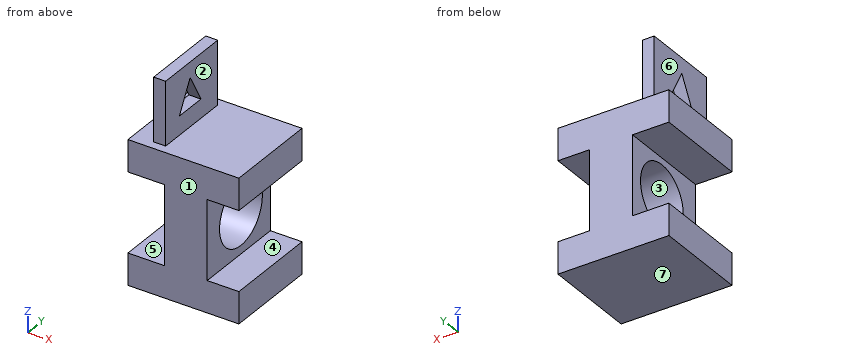
```python
from build123d import *

# Parameters (mm, degrees)
F1_DEPTH = 76.2
F2_W     = 9.595008567
F2_H     = 62.8318372183
F3_DEPTH = 50.8
F5_DEPTH = 25.5704986105
F6_R     = 25.7972308172
F7_DEPTH = 59.7263876276


with BuildPart() as f1:
    # F0 (on Front) → F1 (new body)
    with BuildSketch(Plane.XZ):
        Polygon((-44.6047578722, -25.4), (-44.6047578722, -50.8), (44.2952421278, -50.8), (44.2952421278, -25.4), (18.8952421278, -25.4), (18.8952421278, 38.1), (44.2952421278, 38.1), (44.2952421278, 63.5), (-44.6047578722, 63.5), (-44.6047578722, 38.1), (-15.4301454999, 38.1), (-15.4301454999, -25.4), align=None)
    extrude(amount=F1_DEPTH)

    # F2 (on face) → F3 (join)
    with BuildSketch(Plane.XY.offset(63.5)):
        with Locations((-23.8327635452, -37.7904830966)):
            Rectangle(F2_W, F2_H)
    extrude(amount=F3_DEPTH)

    # F4 (on face) → F5 (cut, through all)
    with BuildSketch(Plane.YZ.offset(-19.0352592617)):
        Polygon((-52.6472702622, 78.5312056541), (-26.647888124, 78.5312056541), (-39.6475791931, 102.0544543862), align=None)
    extrude(amount=-F5_DEPTH, mode=Mode.SUBTRACT)

    # F6 (on face) → F7 (cut, through all)
    with BuildSketch(Plane(origin=(-15.4301454999, 0, 0), x_dir=(0, -1, 0), z_dir=(-1, 0, 0))):
        with Locations((35.4866050184, 7.0887273178)):
            Circle(F6_R)
    extrude(amount=-F7_DEPTH, mode=Mode.SUBTRACT)


solid = f1.part
```
Could you check a few things on this model? Use its own coordinates, in mm. Face numbers are marked on the shaded views. A direction names the side the tool comes from. Coordinates: 2 decimals unless noted, no trailing zeros. Order: outer loops, then holes, each group sorted by start corner. A loop starts at its lowest first (then second) coordinate and runs counter-clockwise, first axis right, second up. Notation, with made-up numbers: M -35.75,-40 L -6.75,-40 A27 ccw -6.75,-19 Z; hole C -25.5,82 d3. An arc over 180 degrees is marked long. Use a Markdown table: item, result. Add a question column.
Q1. I want a section at A-A on x = -24. List the corners of the cut face in (y, z) for me, then the cut area to 3 significant figures.
Q2. I want a section at D-D on y = -42.5. List the corners of the cut face in (x, z) for me, then the cut area to 3 significant figures.
Q3. If I drill on L1, parallel to Z at x = -31, y = -57; L2, parallel to Z at x = -2.5, y = -36; L3, parallel to X at y = -44.5, z = 33.5, over which ranges is the centre line in solid material (lowest first)?
Q4. Which directions (+Z, -Z, +X, -X, +Y, -Y) give clear straight access to the entire face, cutting with the end or side of a thin tool? Please do the marked faces 4, 5, 6 and 7.
Q5. I want a section at C-C on z = 21.5. List the corners of the cut face in (x, y) for me, then the cut area to 3 significant figures.
Q6. I want a section at B-B on x = 25. List the corners of the cut face in (y, z) for me.
Q7. I'm going to push flat-ended pins straight in: pin 1 (6 mm diameter, centred on y = -25, z = -22, fed in from -X); pin 2 (1 mm diameter, centred on x = 21, y = -29.5, fed in from +Z); pin 3 (10.5 mm diameter, centred on x = -24, z = 88.5, fed in from +Y). Where does each tip first touch, or does it pass through?
Q8. We'd pull the mould along Y, two halves only. Please class the marked faces 1, 2 and 3: pulls with the +Y half, pulls with the -Y half, needs draft (parallel to the pull), parting line crosses it, or undercut.
Checked values:
| question | item | result |
|---|---|---|
| 1 | outline | M -76.2,-50.8 L 0,-50.8 L 0,-25.4 L -76.2,-25.4 Z; M -76.2,38.1 L 0,38.1 L 0,63.5 L -6.37,63.5 L -6.37,114.3 L -69.21,114.3 L -69.21,63.5 L -76.2,63.5 Z; hole M -52.65,78.53 L -26.65,78.53 L -39.65,102.05 Z |
| 1 | area | 6,760 mm² |
| 2 | outline | M -44.6,-50.8 L 44.3,-50.8 L 44.3,-25.4 L 18.9,-25.4 L 18.9,-17.74 L -15.43,-17.74 L -15.43,-25.4 L -44.6,-25.4 Z; M -44.6,38.1 L -15.43,38.1 L -15.43,31.91 L 18.9,31.91 L 18.9,38.1 L 44.3,38.1 L 44.3,63.5 L -19.04,63.5 L -19.04,78.53 L -28.63,78.53 L -28.63,63.5 L -44.6,63.5 Z; M -28.63,96.89 L -19.04,96.89 L -19.04,114.3 L -28.63,114.3 Z |
| 2 | area | 5,300 mm² |
| 3 | L1 | -50.8 to -25.4, 38.1 to 63.5 |
| 3 | L2 | -50.8 to -18.7, 32.88 to 63.5 |
| 3 | L3 | -15.43 to 18.9 |
| 4 | face 4 | +X, +Y, -Y |
| 4 | face 5 | -X, +Y, -Y |
| 4 | face 6 | +Z, -X, +Y, -Y |
| 4 | face 7 | -Z, +X, -X, +Y, -Y |
| 5 | outline | M -15.43,-76.2 L 18.9,-76.2 L 18.9,-56.88 L -15.43,-56.88 Z; M -15.43,-14.09 L 18.9,-14.09 L 18.9,0 L -15.43,0 Z |
| 5 | area | 1,150 mm² |
| 6 | outline | M -76.2,-50.8 L 0,-50.8 L 0,-25.4 L -76.2,-25.4 Z; M -76.2,38.1 L 0,38.1 L 0,63.5 L -76.2,63.5 Z |
| 7 | pin 1 | x = -15.43 |
| 7 | pin 2 | z = 63.5 |
| 7 | pin 3 | y = -6.37 |
| 8 | face 1 | pulls with the -Y half |
| 8 | face 2 | needs draft |
| 8 | face 3 | undercut |
